Build history of the part. All positions in model axes, mm. Face numbers are marked on the shaded views. A direction names the side the tool comes from. Round coordinates to 2 decimals unless told otherwise and drop trailing zeros. Write each loop counter-clockwise with the first axis right and the second up, starting at its lowest first coordinate (ties: lowest second). Pieces come first, ordered by that corner, then holes.
1) Wall check: probe 1 along X at (y, z) = (-6, -2); probe 2 along Z at (x, y) = (12, 0); probe 3 along Z at (x, y) = (3.25, 0). Give the ranges that are in metal, low to high.
2) Saw through at A-A (y = 0). Write the cut outline in (x, z), plus the area to 4 significant figures.
3) Flat gauge pins, fed straight in: pin 1 (5 mm diameter, centred on x = 4, z = -4.5, fed in from +Y); pin 2 (1.5 mm diameter, centred on x = 2, z = -5.5, fed in from +Y); pin 3 (4 mm diameter, centred on x = 5.5, y = 5, fed in from +Z); pin 4 (4 mm diameter, centred on y = -0.5, z = 2, fed in from +X). Where does each tip first touch, or does it go through?
4) Saw through at C-C (x = 14.5). Write the cut outline in (y, z).
5) Saw through at D-D (y = -5). Write the cut outline in (x, z), plus the area to 3 significant figures.
6) Which spindle directions (+Z, -Z, +X, -X, +Y, -Y) get a long thin tool onto all of the face, cutting with end or side? Do the marked faces 5 and 6. Say none if no direction does.
7) Pull direction Y, two halves, no side cores. Call the marked faces 1, 2, 3 and 4: +Y half, -Y half, draft (parallel to the pull), parting line (faces both ways), or undercut.
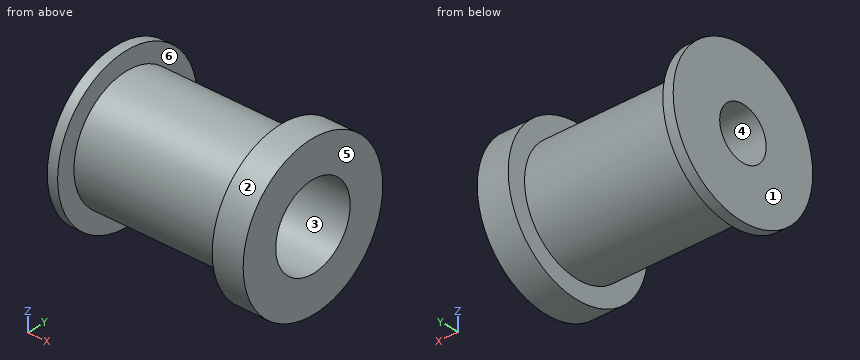
Autodesk Inventor part; units mm, degrees
ref_plane "YZ Plane" through (0, 0, 0) normal (1, 0, 0) x (0, 1, 0)
ref_plane "XZ Plane" through (0, 0, 0) normal (0, 1, 0) x (-1, 0, 0)
ref_plane "XY Plane" through (0, 0, 0) normal (0, 0, 1) x (1, 0, 0)
sketch "Sketch1" plane through (0, 0, 0) normal (0, 0, 1) x (1, 0, 0)
  line L0 (0, 0) -> (4, 0)
  line L1 (0, 0) -> (0, 2.5)
  line L2 (0, 5.75) -> (15, 5.75)
  line L3 (15, 5.75) -> (15, 7.5)
  line L4 (18, 5) -> (18, 4)
  line L5 (18, 4) -> (6, 4)
  line L6 (6, 4) -> (6, 2.5)
  line L7 (6, 2.5) -> (0, 2.5)
  line L8 (0, 5.75) -> (0, 7.5)
  line L9 (0, 7.5) -> (-1, 7.5)
  line L10 (-1, 7.5) -> (-1, 2.5)
  line L11 (-1, 2.5) -> (0, 2.5)
  line L12 (15, 7.5) -> (18, 7.5)
  line L13 (18, 7.5) -> (18, 5)
  dimension "d0" = 4
  dimension "d1" = 5.75
  dimension "d2" = 15
  dimension "d3" = 1.75
  dimension "d7" = 1
  dimension "d8" = 12
  dimension "d9" = 1.5
  dimension "d11" = 1
revolve "Revolution1" add sketch "Sketch1" angle 360 about axis through (0, 0, 0) along (1, 0, 0)
properties part number "pignon 12 dents cournt"
Evaluation:
1. probe 1: x = -1 to 0, 15 to 18
1. probe 2: z = -5.75 to -4, 4 to 5.75
1. probe 3: z = -5.75 to -2.5, 2.5 to 5.75
2. outline: (-1, -7.5) - (0, -7.5) - (0, -5.75) - (15, -5.75) - (15, -7.5) - (18, -7.5) - (18, -4) - (6, -4) - (6, -2.5) - (-1, -2.5) - close; (-1, 2.5) - (6, 2.5) - (6, 4) - (18, 4) - (18, 7.5) - (15, 7.5) - (15, 5.75) - (0, 5.75) - (0, 7.5) - (-1, 7.5) - close
2. area: 101.5 mm2
3. pin 1: stops at y = 5.39
3. pin 2: stops at y = 3.24
3. pin 3: stops at z = 4.91
3. pin 4: stops at x = 18
4. outline: circle Ø11.5 at (0, 0); hole circle Ø8 at (0, 0)
5. outline: (-1, -5.59) - (0, -5.59) - (0, -2.84) - (15, -2.84) - (15, -5.59) - (18, -5.59) - (18, 5.59) - (15, 5.59) - (15, 2.84) - (0, 2.84) - (0, 5.59) - (-1, 5.59) - close
5. area: 130 mm2
6. face 5: +Z, -Z, +X, +Y, -Y
6. face 6: none
7. face 1: draft
7. face 2: parting line
7. face 3: undercut
7. face 4: undercut
